Input: part model. Units: mm. Frame: model coordinates. Face numbers are marked on the shaded views. A direction names the side the tool comes from. Give positions to 0.01 mm unless a question says otherwise; leave off trailing zeros. Loops run counter-clockwise (first coordinate to the right, second up) from the corner with the lowest first, then second, coordinate; pieces in that order, holes last. Notation, with made-up numbers: M 25.25,-5.75 L 42.25,-5.75 A15 cw 42.25,14.25 Z; hole C 3,26.25 d6. An arc over 180 degrees is marked long. Return JSON: item names as keys, results as strings. Group by question number.
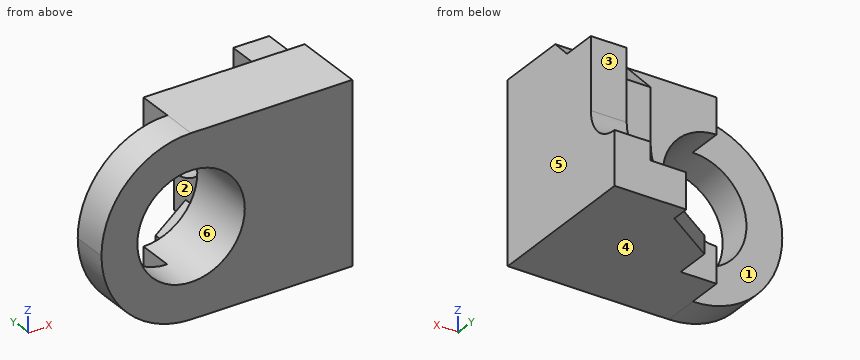
```python
from build123d import *

# Parameters (mm, degrees)
SKETCH2_W           = 140
SKETCH2_H           = 100
BOSS_EXTRUDE2_DEPTH = 90
CUT_EXTRUDE1_DEPTH  = 90
SKETCH4_R           = 30
CUT_EXTRUDE2_DEPTH  = 90
SKETCH5_W           = 50
SKETCH5_H           = 100
CUT_EXTRUDE3_DEPTH  = 90
SKETCH6_W           = 50
SKETCH6_H           = 100
CUT_EXTRUDE4_DEPTH  = 90
CUT_EXTRUDE5_DEPTH  = 20
CUT_EXTRUDE6_DEPTH  = 20
CUT_EXTRUDE7_DEPTH  = 20
BOSS_EXTRUDE3_DEPTH = 10


with BuildPart() as part:
    # Sketch2 → Boss-Extrude2 (new body)
    with BuildSketch(Plane(origin=(0, 0, 0), x_dir=(1, 0, 0), z_dir=(0, 1, 0))):
        with Locations((-70, 50)):
            Rectangle(SKETCH2_W, SKETCH2_H)
    extrude(amount=BOSS_EXTRUDE2_DEPTH)

    # Sketch3 → Cut-Extrude1 (cut)
    with BuildSketch(Plane(origin=(0, 90, 0), x_dir=(1, 0, 0), z_dir=(0, 1, 0))):
        with BuildLine():
            ThreePointArc((-140, 50), (-125.355339059, 85.355339059), (-90, 100))
            Line((-90, 100), (-140, 100))
            Line((-140, 100), (-140, 50))
        make_face()
        with BuildLine():
            ThreePointArc((-90, 0), (-125.355339059, 14.644660941), (-140, 50))
            Line((-140, 50), (-140, 0))
            Line((-140, 0), (-90, 0))
        make_face()
    extrude(amount=-CUT_EXTRUDE1_DEPTH, mode=Mode.SUBTRACT)

    # Sketch4 → Cut-Extrude2 (cut)
    with BuildSketch(Plane(origin=(0, 90, 0), x_dir=(1, 0, 0), z_dir=(0, 1, 0))):
        with Locations((-90, 50)):
            Circle(SKETCH4_R)
    extrude(amount=-CUT_EXTRUDE2_DEPTH, mode=Mode.SUBTRACT)

    # Sketch5 → Cut-Extrude3 (cut)
    with BuildSketch(Plane(origin=(0, 20, 0), x_dir=(1, 0, 0), z_dir=(0, 1, 0))):
        with Locations((-115, 50)):
            Rectangle(SKETCH5_W, SKETCH5_H)
    extrude(amount=CUT_EXTRUDE3_DEPTH, mode=Mode.SUBTRACT)

    # Sketch6 → Cut-Extrude4 (cut)
    with BuildSketch(Plane(origin=(0, 40, 0), x_dir=(1, 0, 0), z_dir=(0, 1, 0))):
        with Locations((-65, 50)):
            Rectangle(SKETCH6_W, SKETCH6_H)
    extrude(amount=CUT_EXTRUDE4_DEPTH, mode=Mode.SUBTRACT)

    # Sketch7 → Cut-Extrude5 (cut)
    with BuildSketch(Plane.ZY.offset(40)):
        with BuildLine():
            Line((-50, 60), (0, 60))
            Line((0, 60), (0, 90))
            Line((0, 90), (-80, 90))
            ThreePointArc((-80, 90), (-71.213203436, 68.786796564), (-50, 60))
        make_face()
    extrude(amount=-CUT_EXTRUDE5_DEPTH, mode=Mode.SUBTRACT)

    # Sketch8 → Cut-Extrude6 (cut)
    with BuildSketch(Plane.ZY.offset(40)):
        Polygon((0, 40), (-20, 60), (0, 60), align=None)
    extrude(amount=-CUT_EXTRUDE6_DEPTH, mode=Mode.SUBTRACT)

    # Sketch9 → Cut-Extrude7 (cut)
    with BuildSketch(Plane.ZY.offset(20)):
        with BuildLine():
            Line((-50, 70), (-10, 70))
            Line((-10, 70), (-10, 50))
            Line((-10, 50), (0, 40))
            Line((0, 40), (0, 90))
            Line((0, 90), (-70, 90))
            ThreePointArc((-70, 90), (-64.142135624, 75.857864376), (-50, 70))
        make_face()
    extrude(amount=-CUT_EXTRUDE7_DEPTH, mode=Mode.SUBTRACT)

    # Sketch10 → Boss-Extrude3 (add)
    with BuildSketch(Plane(origin=(0, 0, -100), x_dir=(-1, 0, 0), z_dir=(0, 0, -1))):
        Polygon((40, 80), (70, 60), (70, 40), (40, 40), align=None)
    extrude(amount=-BOSS_EXTRUDE3_DEPTH)


solid = part.part
```
Item 1: Section B-B, the plane x = -65. Return loops of the section in (y, z).
Item 2: Section C-C, the plane y = 53.5. Return loops of the section in (x, z).
Item 3: Reachability of the marked faces 1, 2 and 3 from +Z, -Z, +X, -X, +Y, -Y: full face, straight path, thin tool, end or side. Return the list, or none.
Item 4: Material intervals for line 1 (Z direction, x = -90, y = 19.5); line 2 (X direction, y = 10, z = -50); line 3 (Y direction, x = -45, z = -40), sorted ascending. Write a range as from..to.
Item 5: Pull-direction query (Z, two-part tool) for the marked faces 4, 5 and 6; classes: pulls with the +Z half, pulls with the -Z half, needs draft (parallel to the pull), parting line crosses it, or undercut.
Item 6: Section A-A, the plane z = -76. Return loops of the section in (x, y).
Item 7: First-contact query: pin 1 Ø6 at (x, z) = (-26, -36) entering from +Y; pin 2 Ø3 at (y, z) = (48.5, -94) entering from -X; pin 3 Ø22 at (y, z) = (33, -94.5) entering from -X. Flat tips, straight axial feed; report the tip coordinate or a pass-through.
Item 8: Section D-D, the plane x = -14.5. Return loops of the section in (y, z), then the cut area to 3 significant figures.
Answer below:
{
 "1": {"outline": "M 0,-100 L 63.33,-100 L 63.33,-90 L 40,-90 L 40,-66.58 L 0,-66.58 Z; M 0,-33.42 L 40,-33.42 L 40,0 L 0,0 Z"},
 "2": {"outline": "M -70,-100 L 0,-100 L 0,-10 L -20,-10 L -20,-13.5 L -40,-13.5 L -40,-90 L -70,-90 Z"},
 "3": {"face 1": "+Z, -Z, -X, +Y", "face 2": "+Z, -X, +Y", "face 3": "+Z, +X, -X, +Y"},
 "4": {"line 1": "-100..-80, -20..0", "line 2": "-140..-120, -60..0", "line 3": "0..40"},
 "5": {"face 4": "pulls with the -Z half", "face 5": "needs draft", "face 6": "undercut"},
 "6": {"outline": "M -132.71,0 L -104.97,0 L -104.97,20 L -132.71,20 Z; M -75.03,0 L 0,0 L 0,90 L -20,90 L -20,75.03 L -40,75.03 L -40,40 L -75.03,40 Z"},
 "7": {"pin 1": "y = 60", "pin 2": "x = -70", "pin 3": "x = -90"},
 "8": {"outline": "M 0,-100 L 90,-100 L 90,-70 A20 cw 70,-50 L 70,-10 L 50,-10 L 40,0 L 0,0 Z", "area": "7,440 mm^2"}
}
